Check sheet for the modelled part. Datum: model origin and axes. Units: mm. Face numbers are marked on the shaded views. A direction names the side the tool comes from. Give positions to 0.01 mm unless a question says otherwise; leave off trailing zeros. Write each loop counter-clockwise with the first axis right and the second up, starting at its lowest first coordinate (ties: lowest second). Pieces come first, ordered by that corner, then holes. Notation, with made-up numbers: (-17.75, 43.5) -> (-3.75, 43.5) arc R18 cw to (-3.75, 61.5) -> close; hole circle Ø1 at (60.5, 49). An arc over 180 degrees is marked (long way). Write each question's results on one line, items separated by ' | '. Start each with the question number.
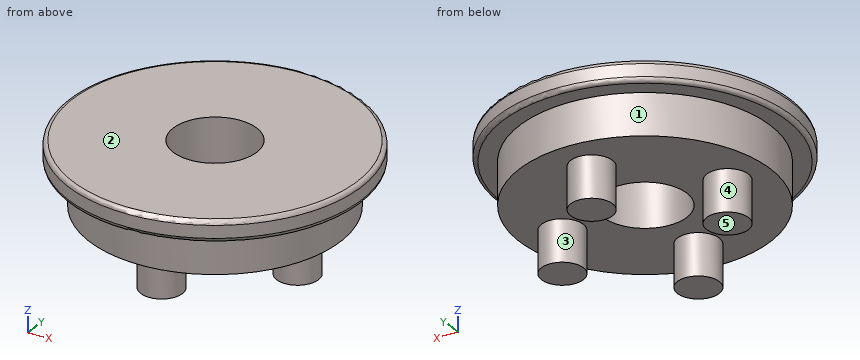
```python
from build123d import *

# Parameters (mm, degrees)
SKETCH1_R           = 35
BOSS_EXTRUDE1_DEPTH = 5
FILLET1_R           = 1
SKETCH2_R           = 30
BOSS_EXTRUDE2_DEPTH = 10
SKETCH3_R           = 5
BOSS_EXTRUDE3_DEPTH = 10
SKETCH4_R           = 10
CUT_EXTRUDE1_DEPTH  = 16


with BuildPart() as part:
    # Sketch1 → Boss-Extrude1 (new body)
    with BuildSketch(Plane.XY):
        Circle(SKETCH1_R)
    extrude(amount=BOSS_EXTRUDE1_DEPTH)

    # Fillet1
    fillet1_edges = [part.edges().sort_by_distance(p)[0] for p in [
        (-35, 0, 0),
        (-35, 0, 5),
    ]]
    fillet(fillet1_edges, radius=FILLET1_R)

    # Sketch2 → Boss-Extrude2 (add)
    with BuildSketch(Plane(origin=(0, 0, 0), x_dir=(-1, 0, 0), z_dir=(0, 0, -1))):
        Circle(SKETCH2_R)
    extrude(amount=BOSS_EXTRUDE2_DEPTH)

    # Sketch3 → Boss-Extrude3 (add)
    with BuildSketch(Plane(origin=(0, 0, -10), x_dir=(-1, 0, 0), z_dir=(0, 0, -1))):
        with Locations((0, 20)):
            Circle(SKETCH3_R)
        with Locations((20, 0)):
            Circle(SKETCH3_R)
        with Locations((0, -20)):
            Circle(SKETCH3_R)
        with Locations((-20, 0)):
            Circle(SKETCH3_R)
    extrude(amount=BOSS_EXTRUDE3_DEPTH)

    # Sketch4 → Cut-Extrude1 (cut, through all)
    with BuildSketch(Plane(origin=(0, 0, -10), x_dir=(-1, 0, 0), z_dir=(0, 0, -1))):
        Circle(SKETCH4_R)
    extrude(amount=-CUT_EXTRUDE1_DEPTH, mode=Mode.SUBTRACT)


solid = part.part
```
Item 1: Section check B-B on z = -14.5. Record the boundary of the cut face in (x, y), then the cut area to 3 significant figures.
Item 2: Depth check by flat-ended pin: pin 1 Ø3 at (x, y) = (-22.5, 9.5) entering from -Z; pin 2 Ø6 at (y, z) = (-8.5, -14) entering from +X; pin 3 Ø6 at (x, z) = (-16.5, -17) entering from -Y; pin 4 Ø8 at (x, z) = (-24.5, -1) entering from -Y. Enter the tip coordinate at first touch or a pass-through.
Item 3: Section check A-A on y = 0. Record the boundary of the cut face in (x, z), then the cut area to 3 significant figures.
Item 4: Set-up check for the marked faces 4 and 5: record each of +Z, -Z, +X, -X, +Y, -Y from which the full face is reachable in a straight line by a thin tool's end or side.
Item 5: Section check C-C on z = -7.25. Record the boundary of the cut face in (x, y).
Item 6: Mould release check, pull along X, two halves, no side actions. Record for the marked faces 1, 2 and 3: pulls with the +X half, pulls with the -X half, needs draft (parallel to the pull), parting line crosses it, or undercut.
Item 7: Thickness scan on probe 1 along Y at (x, z) = (0, -2.5); probe 2 along Y at (x, z) = (0, 1); probe 3 along Z at (x, y) = (-26, 11). Record the ranges inside material, lowest first. Write a range as from..to.
Check sheet entries:
1) outline: circle Ø10 at (-20, 0); circle Ø10 at (0, -20); circle Ø10 at (0, 20); circle Ø10 at (20, 0) | area: 314 mm^2
2) pin 1: stops at z = -10 | pin 2: passes through | pin 3: stops at y = -4.97 | pin 4: stops at y = -28.03
3) outline: (-35, 1) arc R1 ccw to (-34, 0) -> (-30, 0) -> (-30, -10) -> (-25, -10) -> (-25, -20) -> (-15, -20) -> (-15, -10) -> (-10, -10) -> (-10, 5) -> (-34, 5) arc R1 ccw to (-35, 4) -> close; (10, -10) -> (15, -10) -> (15, -20) -> (25, -20) -> (25, -10) -> (30, -10) -> (30, 0) -> (34, 0) arc R1 ccw to (35, 1) -> (35, 4) arc R1 ccw to (34, 5) -> (10, 5) -> close | area: 849 mm^2
4) face 4: -Z | face 5: -Z, +X, -X, +Y, -Y
5) outline: circle Ø60 at (0, 0); hole circle Ø20 at (0, 0)
6) face 1: parting line crosses it | face 2: needs draft | face 3: undercut
7) probe 1: y = -30..-10, 10..30 | probe 2: y = -35..-10, 10..35 | probe 3: z = -10..5
